```python
from build123d import *

# Parameters (mm, degrees)
F0_R     = 4.85
F1_DEPTH = 11
F2_W     = 20
F2_H     = 40
F3_DEPTH = 4
F4_W     = 9
F4_H     = 40
F5_DEPTH = 1.5
F6_SIZE  = 1.49999
F7_R     = 2.75
F8_DEPTH = 31.501


# Not quite as in the source:
# - a fillet or chamfer is up to 0.001 mm smaller than in the source, because OpenCascade refuses the exact size


with BuildPart() as f1:
    # F0 (on Top) → F1 (new body)
    with BuildSketch(Plane.XY):
        Polygon((5.7735026919, 10), (-5.7735026919, 10), (-14.4529946162, 10), (-14.4529946162, -10), (-5.7735026919, -10), (5.7735026919, -10), (11.5470053838, 0), align=None)
        Circle(F0_R, mode=Mode.SUBTRACT)
    extrude(amount=F1_DEPTH)

    # F2 (on face) → F3 (join)
    with BuildSketch(Plane(origin=(-14.4529946162, 0, 0), x_dir=(0, -1, 0), z_dir=(-1, 0, 0))):
        with Locations((0, 5)):
            Rectangle(F2_W, F2_H)
    extrude(amount=F3_DEPTH)

    # F4 (on face) → F5 (join)
    with BuildSketch(Plane(origin=(-18.4529946162, 0, 0), x_dir=(0, -1, 0), z_dir=(-1, 0, 0))):
        with Locations((0, 5)):
            Rectangle(F4_W, F4_H)
    extrude(amount=F5_DEPTH)

    # F6 (size 1.5 in the source; OpenCascade refuses exactly that, so slightly less here)
    f6_edges = [f1.edges().sort_by_distance(p)[0] for p in [
        (-19.952995, 0, 25),
        (-19.952995, 4.5, 5),
        (-19.952995, 0, -15),
        (-19.952995, -4.5, 5),
    ]]
    chamfer(f6_edges, length=F6_SIZE)

    # F7 (on face) → F8 (cut, through all)
    with BuildSketch(Plane(origin=(-19.9529946162, 0, 0), x_dir=(0, -1, 0), z_dir=(-1, 0, 0))):
        with Locations((0, 15)):
            Circle(F7_R)
        with Locations((0, -5)):
            Circle(F7_R)
    extrude(amount=-F8_DEPTH, mode=Mode.SUBTRACT)


solid = f1.part
```
Geometry: final body of the model. Coordinates: model frame, mm. A direction names the side the tool comes from. Coordinates: 2 decimals unless noted, no trailing zeros. Order: outer loops, then holes, each group sorted by start corner. A loop starts at its lowest first (then second) coordinate and runs counter-clockwise, first axis right, second up.
Item 1: Section query A-A (x = 0). Output: boundary loops of the cut face in (y, z), then the cut area to 3 significant figures.
Answer:
outline: (-10, 0) - (-4.85, 0) - (-4.85, 11) - (-10, 11) - close; (4.85, 0) - (10, 0) - (10, 11) - (4.85, 11) - close
area: 113 mm2
Item 2: Contact query for flat-ended pins moving along their axis: P1, Ø3, axis at y = -7, z = 12.5, coming from the -X side; P2, Ø5, axis at y = 0, z = 15, coming from the +X side; P3, Ø1, axis at x = -7.5, y = 2, coming from the -Z side; P4, Ø1, axis at x = -3, y = 4, coming from the +Z side. Output: stop coordinate, or through.
Answer:
P1: stops at x = -18.45
P2: passes through
P3: stops at z = 0
P4: stops at z = 11
Item 3: Access query for faces 1 (the face through (-14.453, 0, 18)), 2 (the face through (-14.453, 0, -9)), 3 (the face through (-18.453, 7, 5)). Directions: +Z, -Z, +X, -X, +Y, -Y. A direction counts if a zero-diameter tool reaches every point of the face in a straight line with its end or side. Return the directions, or none.
Answer:
face 1: +Z, +X, +Y, -Y
face 2: -Z, +X, +Y, -Y
face 3: +Z, -Z, -X, +Y
Item 4: Material intervals for line 1 along Z through (x, y) = (-18.3, 0); line 2 along Y through (x, z) = (4, 7); line 3 along Y through (x, z) = (0, 7.5), sorted ascending.
Answer:
line 1: z = -15 to -7.75, -2.25 to 12.25, 17.75 to 25
line 2: y = -10 to -2.74, 2.74 to 10
line 3: y = -10 to -4.85, 4.85 to 10
Item 5: Draft query along Y for faces 4 (the face through (-17.241, 0.596, -7.685)), 5 (the face through (-5, 2, 11)), 6 (the face through (-9, -10, 5)), 7 (the face through (-17.241, 0.358, 17.727)). Return one class per face: released by +Y, released by -Y, zero draft, split by the parting line, or undercut.
Answer:
face 4: undercut
face 5: zero draft
face 6: released by -Y
face 7: undercut
Item 6: Section query C-C (y = 3.5). Output: boundary loops of the cut face in (x, z), then the cut area to 3 significant figures.
Answer:
outline: (-19.45, -14) - (-18.45, -15) - (-14.45, -15) - (-14.45, 0) - (-3.36, 0) - (-3.36, 11) - (-14.45, 11) - (-14.45, 25) - (-18.45, 25) - (-19.45, 24) - close; (3.36, 0) - (9.53, 0) - (9.53, 11) - (3.36, 11) - close
area: 389 mm2
Item 7: Section query D-D (y = -2.25). Output: boundary loops of the cut face in (x, z).
Answer:
outline: (-19.95, -13.5) - (-18.45, -15) - (-14.45, -15) - (-14.45, -6.58) - (-19.95, -6.58) - close; (-19.95, -3.42) - (-14.45, -3.42) - (-14.45, 0) - (-4.3, 0) - (-4.3, 11) - (-14.45, 11) - (-14.45, 13.42) - (-19.95, 13.42) - close; (-19.95, 16.58) - (-14.45, 16.58) - (-14.45, 25) - (-18.45, 25) - (-19.95, 23.5) - close; (4.3, 0) - (10.25, 0) - (10.25, 11) - (4.3, 11) - close
